Verification items for the finished model (mm, model axes). Coordinates: 2 decimals unless noted, no trailing zeros. Loops run counter-clockwise (first coordinate to the right, second up) from the corner with the lowest first, then second, coordinate; pieces in that order, holes last. Notation, with made-up numbers: (-35, 22.25) -> (17, 22.25) arc R21 cw to (17, 33.25) -> close; hole circle Ø11 at (-23, 56.5). An arc over 180 degrees is marked (long way). Write item = value, one per line.
```python
from build123d import *

# Parameters (mm, degrees)
F0_W     = 482.6
F0_H     = 132.6
F1_DEPTH = 3
F2_W     = 3.5
F2_H     = 6.8
F3_W     = 3.5
F3_H     = 6.8
F4_W     = 3.5
F4_H     = 6.8
F5_W     = 3.5
F5_H     = 6.8
F6_DEPTH = 3
F7_R     = 32
F7_R_2   = 25.5
F7_W     = 64.5
F7_H     = 9
F7_R_3   = 1.9
F8_DEPTH = 3


with BuildPart() as f1:
    # F0 (on Front) → F1 (new body)
    with BuildSketch(Plane.XZ):
        Rectangle(F0_W, F0_H)
    extrude(amount=-F1_DEPTH)

    # F2 (on face) + F3 (on face) + F4 (on face) + F5 (on face) → F6 (cut)
    with BuildSketch(Plane.XZ):
        with Locations((-232.5, 28.6)):
            Rectangle(F2_W, F2_H)
        with BuildLine():
            Line((-230.75, 32), (-230.75, 25.2))
            ThreePointArc((-230.75, 25.2), (-227.35, 28.6), (-230.75, 32))
        make_face()
        with BuildLine():
            ThreePointArc((-234.25, 32), (-237.65, 28.6), (-234.25, 25.2))
            Line((-234.25, 25.2), (-234.25, 32))
        make_face()
    with BuildSketch(Plane.XZ):
        with Locations((-232.5, -28.6)):
            Rectangle(F3_W, F3_H)
        with BuildLine():
            Line((-230.75, -25.2), (-230.75, -32))
            ThreePointArc((-230.75, -32), (-227.35, -28.6), (-230.75, -25.2))
        make_face()
        with BuildLine():
            ThreePointArc((-234.25, -25.2), (-237.65, -28.6), (-234.25, -32))
            Line((-234.25, -32), (-234.25, -25.2))
        make_face()
    with BuildSketch(Plane.XZ):
        with Locations((232.5, 28.6)):
            Rectangle(F4_W, F4_H)
        with BuildLine():
            ThreePointArc((234.25, 25.2), (237.65, 28.6), (234.25, 32))
            Line((234.25, 32), (234.25, 25.2))
        make_face()
        with BuildLine():
            Line((230.75, 25.2), (230.75, 32))
            ThreePointArc((230.75, 32), (227.35, 28.6), (230.75, 25.2))
        make_face()
    with BuildSketch(Plane.XZ):
        with Locations((232.5, -28.6)):
            Rectangle(F5_W, F5_H)
        with BuildLine():
            Line((234.25, -25.2), (234.25, -32))
            ThreePointArc((234.25, -32), (237.65, -28.6), (234.25, -25.2))
        make_face()
        with BuildLine():
            ThreePointArc((230.75, -25.2), (227.35, -28.6), (230.75, -32))
            Line((230.75, -32), (230.75, -25.2))
        make_face()
    extrude(amount=-F6_DEPTH, mode=Mode.SUBTRACT)

    # F7 (on face) → F8 (cut)
    with BuildSketch(Plane.XZ):
        with Locations((-120, 0)):
            Circle(F7_R)
        with Locations((120, 0)):
            Circle(F7_R_2)
        Rectangle(F7_W, F7_H)
        with Locations((38.85, 0)):
            Circle(F7_R_3)
        with Locations((-38.85, 0)):
            Circle(F7_R_3)
    extrude(amount=-F8_DEPTH, mode=Mode.SUBTRACT)


solid = f1.part
```
1) Sectioned sample at A-A, the plane y = 0.5. Count the separate pieces of the cut face and the enclosed holes in it, plus the area to 3 significant figures.
Ans:
separate_pieces = 1
enclosed_holes = 9
area = 57,900 mm2
2) Sectioned sample at B-B, the plane x = -17.5. Record the cut outline in (y, z), plus the area to 3 significant figures.
Ans:
outline = (0, -66.3) -> (3, -66.3) -> (3, -4.5) -> (0, -4.5) -> close; (0, 4.5) -> (3, 4.5) -> (3, 66.3) -> (0, 66.3) -> close
area = 371 mm2
3) Material ranges on line 1 (Z direction, x = 38.85, y = 0.8); line 2 (X direction, y = 0.35, z = -7); line 3 (Z direction, x = -122.5, y = 2.8), recorded low to high.
Ans:
line_1 = -66.3 to -1.9, 1.9 to 66.3
line_2 = -241.3 to -151.22, -88.78 to 95.48, 144.52 to 241.3
line_3 = -66.3 to -31.9, 31.9 to 66.3
4) Release check for a two-part mould opening along Z. For faces 1 (the face through (99.764, 1.479, -15.516)), 2 (the face through (-3, 3, 16)), 3 (the face through (-151.97, 1.48, 1.41)) record: pulls with the +Z half, pulls with the -Z half, needs draft (parallel to the pull), parting line crosses it, or undercut.
Ans:
face_1 = undercut
face_2 = needs draft
face_3 = undercut
